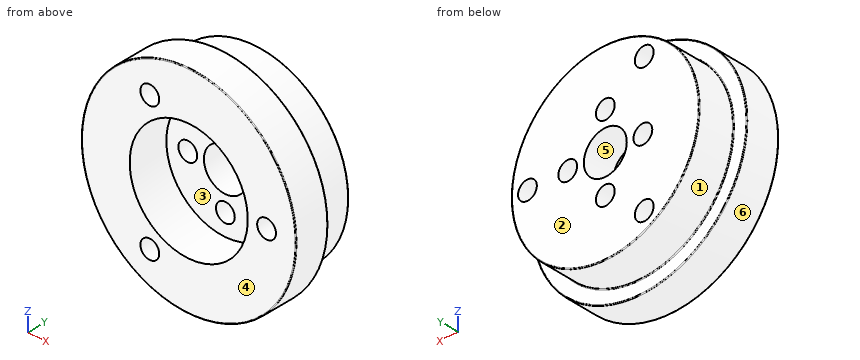
```python
from build123d import *

# Parameters (mm, degrees)
SKETCH2_R          = 1.75
SKETCH2_R_2        = 4
CUT_EXTRUDE4_DEPTH = 32.340867888
SKETCH7_R          = 11
CUT_EXTRUDE5_DEPTH = 7.5
FILLET1_R          = 0.15


with BuildPart() as part:
    # Sketch1 → Revolve1 (revolve)
    with BuildSketch(Plane.XY):
        Polygon((0, 0), (-20, 0), (-20, 6.5), (-17.5, 6.5), (-17.5, 13.5), (0, 13.5), align=None)
    revolve(axis=Axis((0, 13.5, 0), (0, -1, 0)))

    # Sketch2 → Cut-Extrude4 (cut, through all)
    with BuildSketch(Plane.XZ):
        with Locations(Location((-7.25, 12.557368355, 0), (0, 0, 270))):
            Circle(SKETCH2_R)
        with Locations(Location((-7.25, -12.557368355, 0), (0, 0, 270))):
            Circle(SKETCH2_R)
        with Locations(Location((14.5, 0, 0), (0, 0, 270))):
            Circle(SKETCH2_R)
        with Locations(Location((7, 0, 0), (0, 0, 270))):
            Circle(SKETCH2_R)
        with Locations(Location((0, -7, 0), (0, 0, 270))):
            Circle(SKETCH2_R)
        with Locations(Location((-7, 0, 0), (0, 0, 270))):
            Circle(SKETCH2_R)
        with Locations(Location((0, 7, 0), (0, 0, 270))):
            Circle(SKETCH2_R)
        with Locations(Location((0, 0, 0), (0, 0, 270))):
            Circle(SKETCH2_R_2)
    extrude(amount=-CUT_EXTRUDE4_DEPTH, mode=Mode.SUBTRACT)

    # Sketch7 → Cut-Extrude5 (cut)
    with BuildSketch(Plane.XZ):
        with Locations(Location((0, 0, 0), (0, 0, 270))):
            Circle(SKETCH7_R)
    extrude(amount=-CUT_EXTRUDE5_DEPTH, mode=Mode.SUBTRACT)

    # Fillet1
    fillet1_edges = [part.edges().sort_by_distance(p)[0] for p in [
        (17.5, 13.5, 0),
        (17.5, 6.5, 0),
        (20, 6.5, 0),
        (20, 0, 0),
    ]]
    fillet(fillet1_edges, radius=FILLET1_R)


solid = part.part
```
Design review of the part built by this model. Coordinates are the model's own, in mm. Face numbers are marked on the shaded views. A direction names the side the tool comes from. Give positions to 0.01 mm unless a question says otherwise; leave off trailing zeros. Use a Markdown table: item, result. Add a question column.
(1) Machinability: for the marked faces 1, 2 and 3, which of the approach directions +Z, -Z, +X, -X, +Y, -Y give a long, thin tool a straight path to every point of the face, cutting with its end or side? Answer none if there is none.
(2) Clearance check with flat-ended pins moving along their axes: P1, Ø13, axis at x = 0, z = 0, coming from the -Y side; P2, Ø2, axis at x = 0, z = -7, coming from the -Y side; P3, Ø6, axis at y = 7.5, z = 5.5, coming from the +X side; P4, Ø5, axis at y = 11.5, z = -15, coming from the +X side. State where each tip first meets the part, or that it passes through.
(3) Add section A-A on y = 12.75. Give the number of separate pieces and of enclosed holes in the cut face, then the cut area to 4 significant figures.
(4) Mouldability with a two-part tool opening along Z and no side actions: class the marked faces 4, 5 and 6 as +Z half, -Z half, draft (parallel to the pull), parting line (faces both ways), or undercut.
(5) Wall thickness on probe 1 along X at (y, z) = (6, 0); probe 2 along Z at (x, y) = (-1, 8); probe 3 along X at (y, z) = (2.5, 1.5): over which ranges is each line inside the solid? List them lowest first. Write a range as [from, to].
Report:
| question | item | result |
|---|---|---|
| 1 | face 1 | +Y |
| 1 | face 2 | +Z, -Z, +X, -X, +Y |
| 1 | face 3 | -Y |
| 2 | P1 | stops at y = 7.5 |
| 2 | P2 | passes through |
| 2 | P3 | stops at x = 19.81 |
| 2 | P4 | stops at x = 12.25 |
| 3 | separate pieces | 1 |
| 3 | enclosed holes | 8 |
| 3 | area | 844.5 mm² |
| 4 | face 4 | draft |
| 4 | face 5 | undercut |
| 4 | face 6 | parting line |
| 5 | probe 1 | x = [-20, -11], [11, 12.75], [16.25, 20] |
| 5 | probe 2 | z = [-17.47, -8.44], [-5.56, -3.87], [3.87, 5.56], [8.44, 17.47] |
| 5 | probe 3 | x = [-19.94, -10.9], [10.9, 13.6], [15.4, 19.94] |
